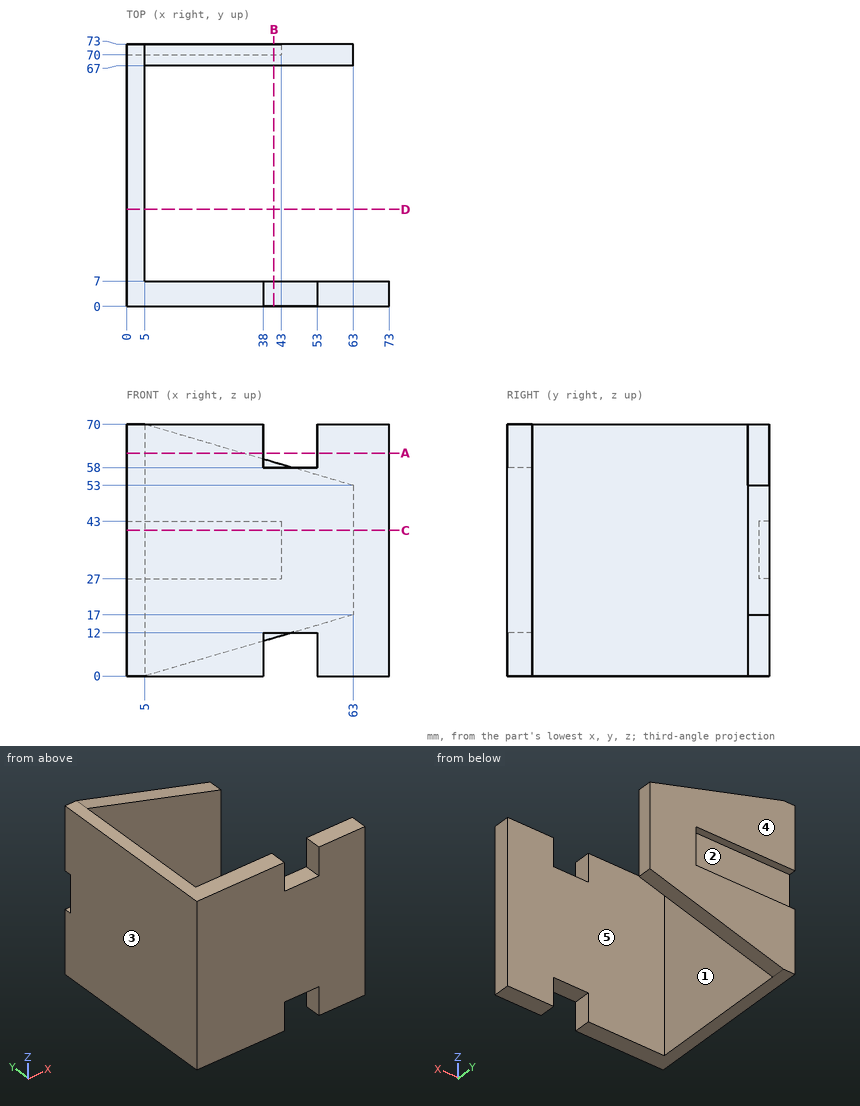
The figure shows three views and two pictorial views of one solid part (mm, origin at its lowest corner). Answer the questions. A direction names the side the tool comes from. Coordinates: 2 decimals unless noted, no trailing zeros. Loops run counter-clockwise (first coordinate to the right, second up) from the corner with the lowest first, then second, coordinate; pieces in that order, holes last. Notation, with made-up numbers: (6.5, -23) -> (10.5, -23) arc R24 ccw to (10.5, 8) -> close; hole circle Ø9 at (78.5, 54). An arc over 180 degrees is marked (long way). Write item = value, one per line. Start each with the question number.
1) Straight lines are drawn through the part: line 1 (Y direction, x = 52.5, z = 56); line 2 (Y direction, x = 11, z = 38.5); line 3 (Z direction, x = 48, y = 3). For each, find the intervals that lie inside material, in ascending order. Write a range as from..to.
2) A cutting plane is placed at B-B (x = 41). Give the vertices of the cut face in (y, z).
3) Given pin 1 Ø3.5 at (x, y) = (46.5, 2) entering from -Z; pin 2 Ø2 at (x, y) = (43, 2) entering from +Z; pin 3 Ø10 at (y, z) = (50, 50) entering from +X; pin 4 Ø10 at (x, y) = (8, 51.5) entering from +Z, each flat-ended and moving along its own axis, determine where each tip first touches the part or whether it passes through.
4) A cutting plane is placed at C-C (z = 40.5). Give the vertices of the cut face in (x, y), then the cut area to 3 significant figures.
5) The mould has two halves that part along Y. Classify the marked faces 1, 2 and 3: released by +Y, released by -Y, zero draft, split by the parting line, or undercut.
6) A cutting plane is placed at A-A (z = 62). Give the vertices of the cut face in (x, y).
7) A tool of negligible diameter and unlimited length cuts with its end or side. For the marked faces 4 and 5, from which of +Z, -Z, +X, -X, +Y, -Y can it reach the whole face along a straight path? Write none if from no direction.
8) A cutting plane is placed at D-D (y = 27). Give the vertices of the cut face in (x, z).
Responses:
q1.line_1 = 0..7, 67..73
q1.line_2 = 0..7, 67..70
q1.line_3 = 12..58
q2.outline = (0, 12) -> (7, 12) -> (7, 58) -> (0, 58) -> close; (67, 10.55) -> (73, 10.55) -> (73, 27) -> (70, 27) -> (70, 43) -> (73, 43) -> (73, 59.45) -> (67, 59.45) -> close
q3.pin_1 = 12
q3.pin_2 = 58
q3.pin_3 = 5
q3.pin_4 = 70
q4.outline = (0, 0) -> (73, 0) -> (73, 7) -> (5, 7) -> (5, 67) -> (63, 67) -> (63, 73) -> (43, 73) -> (43, 70) -> (0, 70) -> close
q4.area = 1,060 mm²
q5.face_1 = undercut
q5.face_2 = released by +Y
q5.face_3 = zero draft
q6.outline = (0, 0) -> (38, 0) -> (38, 7) -> (5, 7) -> (5, 67) -> (32.29, 67) -> (32.29, 73) -> (0, 73) -> close; (53, 0) -> (73, 0) -> (73, 7) -> (53, 7) -> close
q7.face_4 = +Z, -Z, +X, -X, +Y
q7.face_5 = +Z, -Z, +X
q8.outline = (0, 0) -> (5, 0) -> (5, 70) -> (0, 70) -> close
